Part model, mm, in its own coordinate system. Face numbers are marked on the shaded views. A direction names the side the tool comes from. Coordinates: 2 decimals unless noted, no trailing zeros. Loops run counter-clockwise (first coordinate to the right, second up) from the corner with the lowest first, then second, coordinate; pieces in that order, holes last. Notation, with made-up numbers: (52, 31.25) - (62, 31.25) arc R18 ccw to (62, 59.25) - close; hole circle Ø3 at (86.25, 27.5). An arc over 180 degrees is marked (long way). Use a Markdown table: item, result. Add a question column.
1) Band-saw the part on A-A (z = 64). Give the cut face in (x, y) (3 decimals).
2) Band-saw the part on C-C (y = 11.25). Give the cut face in (x, z) (1 decimal).
3) Pull direction Z, two halves, no side cores. Call the marked faces 3 and 4: +Z half, -Z half, draft (parallel to the pull), parting line (faces both ways), or undercut.
4) Drop flat-ended pins along their axis: P1, Ø1, axis at y = -2, z = -29, coming from the +X side (3 decimals); P2, Ø3.5, axis at x = -43, y = -2, coming from the +Z side; P3, Ø3.5, axis at y = -2, z = 22.5, coming from the -X side (3 decimals). Give the stop position or say it passes through.
5) Band-saw the part on D-D (z = -110). Give the cut face in (x, y) (3 decimals), plus the area to 3 significant figures.
6) Band-saw the part on B-B (x = -89). Give the cut face in (y, z) (1 decimal).
7) Probe probe 1 along Z at (x, y) = (-48, 7.5); probe 2 along X at (y, z) = (7.75, 83) (3 decimals); probe 3 along Y at (x, z) = (-34, -116) (3 decimals). List the from-to ranges inside material, lowest first. Write a range as [from, to].
8) Tool access for the marked faces 1 and 2: list every direction of +Z, -Z, +X, -X, +Y, -Y with a clear straight run to the whole face (end or side of a thin tool).
from build123d import *

# Parameters (mm, degrees)
F0_W     = 298.45
F0_H     = 25.4
F0_H_2   = 193.675
F0_W_2   = 285.75
F0_H_3   = 180.975
F1_DEPTH = 3.175
F2_W     = 304.8
F2_H     = 225.425
F2_W_2   = 298.45
F2_H_2   = 219.075
F3_DEPTH = 25.4
F4_SIZE  = 3.81


with BuildPart() as f1:
    # F0 (on Front) → F1 (new body)
    with BuildSketch(Plane.XZ):
        with Locations((0, -109.5375)):
            Rectangle(F0_W, F0_H)
        Rectangle(F0_W, F0_H_2)
        Rectangle(F0_W_2, F0_H_3, mode=Mode.SUBTRACT)
    extrude(amount=F1_DEPTH)

    # F2 (on face) → F3 (join)
    with BuildSketch(Plane.XZ.offset(3.175)):
        with Locations((0, -12.7)):
            Rectangle(F2_W, F2_H)
        with Locations((0, -12.7)):
            Rectangle(F2_W_2, F2_H_2, mode=Mode.SUBTRACT)
    extrude(amount=-F3_DEPTH)

    # F4
    f4_edges = [f1.edges().sort_by_distance(p)[0] for p in [
        (-152.4, -3.175, -12.7),
        (0, -3.175, -125.4125),
        (152.4, -3.175, -12.7),
        (0, -3.175, 100.0125),
    ]]
    chamfer(f4_edges, length=F4_SIZE)


solid = f1.part
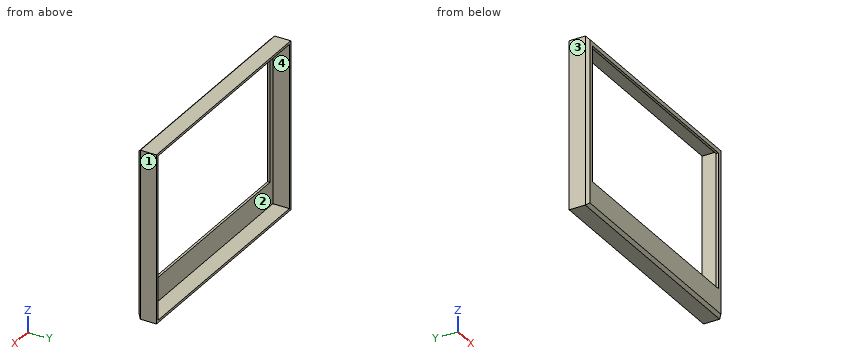
Answer block:
| question | item | result |
|---|---|---|
| 1 | outline | (-152.4, 0.635) - (-148.59, -3.175) - (-142.875, -3.175) - (-142.875, 0) - (-149.225, 0) - (-149.225, 22.225) - (-152.4, 22.225) - close; (142.875, -3.175) - (148.59, -3.175) - (152.4, 0.635) - (152.4, 22.225) - (149.225, 22.225) - (149.225, 0) - (142.875, 0) - close |
| 2 | outline | (-152.4, -125.4) - (152.4, -125.4) - (152.4, 100) - (-152.4, 100) - close; hole (-149.2, -122.2) - (149.2, -122.2) - (149.2, 96.8) - (-149.2, 96.8) - close |
| 3 | face 3 | draft |
| 3 | face 4 | undercut |
| 4 | P1 | x = 150.265 |
| 4 | P2 | z = 99.13 |
| 4 | P3 | x = -151.515 |
| 5 | outline | (-152.4, 0.635) - (-148.59, -3.175) - (148.59, -3.175) - (152.4, 0.635) - (152.4, 22.225) - (149.225, 22.225) - (149.225, 0) - (-149.225, 0) - (-149.225, 22.225) - (-152.4, 22.225) - close |
| 5 | area | 1,090 mm2 |
| 6 | outline | (-3.2, -121.6) - (0.6, -125.4) - (22.2, -125.4) - (22.2, -122.2) - (0, -122.2) - (0, -90.5) - (-3.2, -90.5) - close; (-3.2, 90.5) - (0, 90.5) - (0, 96.8) - (22.2, 96.8) - (22.2, 100) - (0.6, 100) - (-3.2, 96.2) - close |
| 7 | probe 1 | [-125.41, -122.24], [96.84, 100.01] |
| 7 | probe 2 | [-152.4, -149.225], [149.225, 152.4] |
| 7 | probe 3 | [-3.175, 0] |
| 8 | face 1 | +Z, -Z, +X, +Y, -Y |
| 8 | face 2 | +Y |
